from build123d import *

# Parameters (mm, degrees)
F0_W     = 38.1
F0_H     = 38.1
F1_DEPTH = 38.1
F2_DEPTH = 304.8
F3_START = -304.8
F3_DEPTH = 38.1
F4_START = -304.8
F0_W_2   = 50.8
F0_H_2   = 190.5
F4_DEPTH = 38.1
F5_DEPTH = 342.9


with BuildPart() as f1:
    # F0 (on Front) → F1 (new body)
    with BuildSketch(Plane.XZ):
        Polygon((596.9, 38.1), (38.1, 38.1), (38.1, 254), (0, 254), (0, 0), (635, 0), (635, 254), (596.9, 254), align=None)
        with Locations((19.05, 273.05)):
            Rectangle(F0_W, F0_H)
        Polygon((38.1, 292.1), (38.1, 254), (596.9, 254), (596.9, 292.1), (492.125, 292.1), (441.325, 292.1), (193.675, 292.1), (142.875, 292.1), align=None)
        with Locations((615.95, 273.05)):
            Rectangle(F0_W, F0_H)
    extrude(amount=F1_DEPTH)

    # F0 (on Front) → F2 (join)
    with BuildSketch(Plane.XZ):
        with Locations((19.05, 273.05)):
            Rectangle(F0_W, F0_H)
        with Locations((615.95, 273.05)):
            Rectangle(F0_W, F0_H)
    extrude(amount=-F2_DEPTH)

    # F0 (on Front) → F3 (join)
    with BuildSketch(Plane.XZ.offset(F3_START)):
        Polygon((38.1, 292.1), (38.1, 254), (596.9, 254), (596.9, 292.1), (492.125, 292.1), (441.325, 292.1), (193.675, 292.1), (142.875, 292.1), align=None)
        with Locations((19.05, 273.05)):
            Rectangle(F0_W, F0_H)
        with Locations((615.95, 273.05)):
            Rectangle(F0_W, F0_H)
    extrude(amount=-F3_DEPTH)

    # F0 (on Front) → F4 (join)
    with BuildSketch(Plane.XZ.offset(F4_START)):
        with Locations((168.275, 387.35)):
            Rectangle(F0_W_2, F0_H_2)
        with Locations((466.725, 387.35)):
            Rectangle(F0_W_2, F0_H_2)
    extrude(amount=-F4_DEPTH)

    # F0 (on Front) → F5 (join)
    with BuildSketch(Plane.XZ):
        Polygon((117.475, 482.6), (142.875, 482.6), (193.675, 482.6), (193.675, 508), (117.475, 508), align=None)
        Polygon((441.325, 482.6), (492.125, 482.6), (517.525, 482.6), (517.525, 508), (441.325, 508), align=None)
    extrude(amount=-F5_DEPTH)


solid = f1.part
The model under review builds one solid part; all positions refer to its coordinate system, in mm. A direction names the side the tool comes from. Give positions to 0.01 mm unless a question says otherwise; leave off trailing zeros. Order: outer loops, then holes, each group sorted by start corner. A loop starts at its lowest first (then second) coordinate and runs counter-clockwise, first axis right, second up. Notation, with made-up numbers: M 38,-16 L 68,-16 A8 ccw 68,-3 Z; hole C 52.25,5 d10. An arc over 180 degrees is marked long. One line per question, with ' | ' between items. Start each with the question number.
1) Clearance check with flat-ended pins moving along their axes: P1, Ø7.5, axis at x = 493, z = 498.5, coming from the -Y side; P2, Ø12, axis at x = 107.5, y = 164.5, coming from the -Z side; P3, Ø7.5, axis at y = 233.5, z = 494, coming from the +X side (3 decimals); P4, Ø23, axis at x = 496.5, y = 197, coming from the -Z side. State where each tip first meets the part, or that it passes through.
2) Consider section C-C, the plane z = 145. Give the boundary of the cut face in (x, y), then the cut area to 3 significant figures.
3) Consider section D-D, the plane z = 284. Give the boundary of the cut face in (x, y).
4) For faces 5 (the face through (316, 304.8, 284)), 6 (the face through (193.675, 234, 488)), 7 (the face through (596.9, 150, 273)), 8 (the face through (340, 0, 34)), list the 3-axis set-ups (+Z, -Z, +X, -X, +Y, -Y) from which the entire face can be reached by the end or side of a thin tool; tool diameter is ignored.
5) Mouldability with a two-part tool opening along X and no side actions: class faces 1 (the face through (142.875, 324, 386)), 2 (the face through (480, 169, 508)), 3 (the face through (314, 0, 273)), 4 (the face through (321, -19, 38.1)) as pulls with the +X half, pulls with the -X half, needs draft (parallel to the pull), parting line crosses it, or undercut.
6) Consider section A-A, the plane y = 165. Give the boundary of the cut face in (x, z) (3 decimals).
7) Consider section B-B, the plane x = 304.5. Give the boundary of the cut face in (y, z).
8) Wall thickness on L1, parallel to X at y = 109.5, z = 277.5; L2, parallel to Z at x = 31, y = 198.5; L3, parallel to X at y = 305, z = 473 (3 decimals): over which ranges is each line inside the solid? List them lowest first. Write a range as from..to.
Found:
1) P1: stops at y = 0 | P2: passes through | P3: stops at x = 517.525 | P4: stops at z = 482.6
2) outline: M 0,-38.1 L 38.1,-38.1 L 38.1,0 L 0,0 Z; M 596.9,-38.1 L 635,-38.1 L 635,0 L 596.9,0 Z | area: 2,900 mm²
3) outline: M 0,-38.1 L 635,-38.1 L 635,342.9 L 0,342.9 Z; hole M 38.1,0 L 596.9,0 L 596.9,304.8 L 38.1,304.8 Z
4) face 5: -Z | face 6: +Z, +Y, -Y | face 7: +Z, -Z | face 8: -Z, +X, -X, +Y
5) face 1: pulls with the -X half | face 2: needs draft | face 3: undercut | face 4: undercut
6) outline: M 0,254 L 38.1,254 L 38.1,292.1 L 0,292.1 Z; M 117.475,482.6 L 193.675,482.6 L 193.675,508 L 117.475,508 Z; M 441.325,482.6 L 517.525,482.6 L 517.525,508 L 441.325,508 Z; M 596.9,254 L 635,254 L 635,292.1 L 596.9,292.1 Z
7) outline: M -38.1,0 L 0,0 L 0,38.1 L -38.1,38.1 Z; M -38.1,254 L 0,254 L 0,292.1 L -38.1,292.1 Z; M 304.8,254 L 342.9,254 L 342.9,292.1 L 304.8,292.1 Z
8) L1: x = 0..38.1, 596.9..635 | L2: z = 254..292.1 | L3: x = 142.875..193.675, 441.325..492.125
